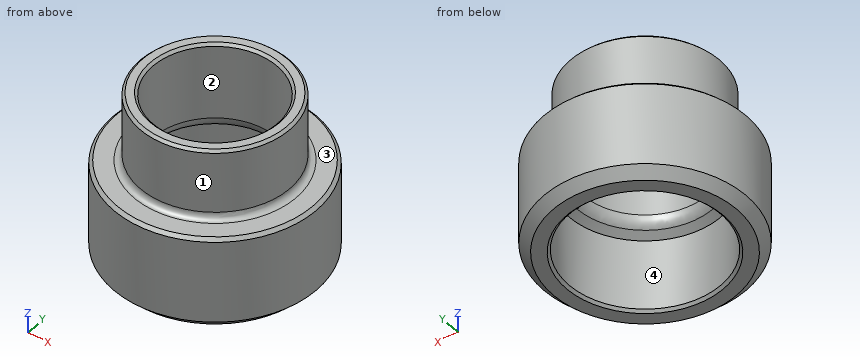
from build123d import *

# Parameters (mm, degrees)
F_12_0_12_DIAMETER_HOLE1_D     = 12
F_12_0_12_DIAMETER_HOLE1_DEPTH = 5.75
F_12_0_12_DIAMETER_HOLE1_TIP   = 3.605163714
CHAMFER1_SIZE                  = 0.75
CHAMFER2_SIZE                  = 0.25
CHAMFER3_SIZE                  = 0.2
FILLET1_R                      = 1


with BuildPart() as part:
    # Sketch1 → Revolve1 (revolve)
    with BuildSketch(Plane.XZ):
        with BuildLine():
            Line((5.9, 13), (4.9, 13))
            Line((4.9, 13), (4.9, 5.75))
            Line((4.9, 5.75), (0, 5.75))
            Line((0, 5.75), (0, 0))
            Line((0, 0), (8, 0))
            Line((8, 0), (8, 7.5))
            Line((8, 7.5), (6.4, 7.5))
            ThreePointArc((6.4, 7.5), (6.046446609, 7.646446609), (5.9, 8))
            Line((5.9, 8), (5.9, 13))
        make_face()
    revolve(axis=Axis((0, 0, 13), (0, 0, -1)))

    # Ø12.0 (12) Diameter Hole1
    with Locations(Plane(origin=(0, 0, 0), x_dir=(-1, 0, 0), z_dir=(0, 0, -1))):
        with Locations((0, 0)):
            Hole(F_12_0_12_DIAMETER_HOLE1_D / 2, depth=F_12_0_12_DIAMETER_HOLE1_DEPTH)
            with Locations((0, 0, -(F_12_0_12_DIAMETER_HOLE1_DEPTH + F_12_0_12_DIAMETER_HOLE1_TIP / 2))):  # 118° drill point
                Cone(0, F_12_0_12_DIAMETER_HOLE1_D / 2, F_12_0_12_DIAMETER_HOLE1_TIP, mode=Mode.SUBTRACT)

    # Chamfer1
    chamfer1_edges = [part.edges().sort_by_distance(p)[0] for p in [
        (-8, 0, 0),
    ]]
    chamfer(chamfer1_edges, length=CHAMFER1_SIZE)

    # Chamfer2
    chamfer2_edges = [part.edges().sort_by_distance(p)[0] for p in [
        (-8, 0, 7.5),
    ]]
    chamfer(chamfer2_edges, length=CHAMFER2_SIZE)

    # Chamfer3
    chamfer3_edges = [part.edges().sort_by_distance(p)[0] for p in [
        (-6, 0, 0),
        (-5.9, 0, 13),
        (-4.9, 0, 13),
    ]]
    chamfer(chamfer3_edges, length=CHAMFER3_SIZE)

    # Fillet1
    fillet1_edges = [part.edges().sort_by_distance(p)[0] for p in [
        (0, -4.9, 6.410946681),
    ]]
    fillet(fillet1_edges, radius=FILLET1_R)


solid = part.part
Work out the finished part from the listing and answer in its coordinate system (mm). Face numbers are marked on the shaded views. Round coordinates to 2 decimals unless told otherwise and drop trailing zeros. Loops run counter-clockwise (first coordinate to the right, second up) from the corner with the lowest first, then second, coordinate; pieces in that order, holes last. Notation, with made-up numbers: (78.5, -3.5) - (131.5, -3.5) arc R18 ccw to (131.5, 8.5) - close; hole circle Ø4 at (49.25, 47). An arc over 180 degrees is marked (long way). Use one line per item in the form item = value. Start each with the question number.
(1) Find section A-A on z = 3.75. Determine the outline of the cut face in (x, y), and give its area (3 significant figures).
(2) Find section B-B on z = 11. Determine the outline of the cut face in (x, y).
(3) Flat-ended cylindrical pins translate along their axes: P1, Ø2, axis at x = -4, z = 3.5, coming from the -Y side; P2, Ø4, axis at y = -6, z = 9, coming from the -X side; P3, Ø3, axis at x = 2, z = 8.5, coming from the -Y side; P4, Ø3, axis at y = -0.5, z = 5.5, coming from the +X side. Find the tip coordinate at first contact, or state that the pin passes through.
(4) Consider line 1 (X direction, y = 0, z = 8.55); line 2 (X direction, y = 0, z = 3.3). Determine where each line is inside the solid, lowest interval first.
(5) Determine the mould class of the marked faces 1, 2, 3 and 4 for opening direction X: +X half, -X half, draft (parallel to the pull), parting line (faces both ways), or undercut.
Answer list:
q1.outline = circle Ø16 at (0, 0); hole circle Ø12 at (0, 0)
q1.area = 88.0 mm^2
q2.outline = circle Ø11.8 at (0, 0); hole circle Ø9.8 at (0, 0)
q3.P1 = -7.42
q3.P2 = -6.22
q3.P3 = -7.91
q3.P4 = 8
q4.line_1 = -5.9 to -4.9, 4.9 to 5.9
q4.line_2 = -8 to -6, 6 to 8
q5.face_1 = parting line
q5.face_2 = undercut
q5.face_3 = draft
q5.face_4 = undercut
